from build123d import *

# Parameters (mm, degrees)
EXTRUDE_1_DEPTH     = 5.5
FILLET_2_R          = 5
SKETCH_5_R          = 0.75
CUT_EXTRUDE_3_DEPTH = 133.967101194
SKETCH_6_R          = 1.05
CUT_EXTRUDE_4_DEPTH = 133.967101194
SKETCH_7_R          = 1.05
CUT_EXTRUDE_5_DEPTH = 133.967101194
FILLET_3_R          = 3
FILLET_4_R          = 10
SKETCH_8_W          = 5.5
SKETCH_8_H          = 5.5
CUT_EXTRUDE_6_DEPTH = 133.967101194
SKETCH_9_R          = 1.05
CUT_EXTRUDE_7_DEPTH = 133.967101194
SKETCH_10_W         = 5.5
SKETCH_10_H         = 100
CUT_EXTRUDE_8_DEPTH = 133.967101194


with BuildPart() as part:
    # ｽｹｯﾁ1 → ﾎﾞｽ - 押し出し1 (new body)
    with BuildSketch(Plane.XY):
        with BuildLine():
            Line((19, 125), (-41, 125))
            Line((-41, 125), (-41, 111))
            Line((-41, 111), (-28, 95))
            Line((-28, 95), (-19, 95))
            Line((-19, 95), (-19, 56.216441442))
            ThreePointArc((-19, 56.216441442), (-31.652114797, 51.899926796), (-45, 51.163538212))
            Line((-45, 51.163538212), (-45, 48.163538212))
            Line((-45, 48.163538212), (-19, 48.163538212))
            Line((-19, 48.163538212), (-19, 23.216373532))
            ThreePointArc((-19, 23.216373532), (0, -30), (19, 23.216373532))
            Line((19, 23.216373532), (19, 125))
        make_face()
    extrude(amount=EXTRUDE_1_DEPTH)

    # ﾌｨﾚｯﾄ2
    fillet_2_edges = [part.edges().sort_by_distance(p)[0] for p in [
        (-19, 95, 2.75),
    ]]
    fillet(fillet_2_edges, radius=FILLET_2_R)

    # ｽｹｯﾁ5 → ｶｯﾄ - 押し出し3 (cut, through all)
    with BuildSketch(Plane.XY.offset(5.5)):
        with Locations((14.45, 0)):
            Circle(SKETCH_5_R)
        with Locations((-14.45, 0)):
            Circle(SKETCH_5_R)
    extrude(amount=-CUT_EXTRUDE_3_DEPTH, mode=Mode.SUBTRACT)

    # ｽｹｯﾁ6 → ｶｯﾄ - 押し出し4 (cut, through all)
    with BuildSketch(Plane.XY.offset(5.5)):
        with Locations((-24.425038206, -12.880897043)):
            Circle(SKETCH_6_R)
        with Locations((-21.701843031, -17.074249883)):
            Circle(SKETCH_6_R)
        with Locations(Location((24.425038206, -12.880897043, 0), (0, 0, 180))):
            Circle(SKETCH_6_R)
        with Locations(Location((21.701843031, -17.074249883, 0), (0, 0, 180))):
            Circle(SKETCH_6_R)
    extrude(amount=-CUT_EXTRUDE_4_DEPTH, mode=Mode.SUBTRACT)

    # ｽｹｯﾁ7 → ｶｯﾄ - 押し出し5 (cut, through all)
    with BuildSketch(Plane.XY.offset(5.5)):
        with Locations((-21.9, 100)):
            Circle(SKETCH_7_R)
        with Locations((-35.6, 110.5)):
            Circle(SKETCH_7_R)
    extrude(amount=-CUT_EXTRUDE_5_DEPTH, mode=Mode.SUBTRACT)

    # ﾌｨﾚｯﾄ3
    fillet_3_edges = [part.edges().sort_by_distance(p)[0] for p in [
        (-28, 95, 2.75),
    ]]
    fillet(fillet_3_edges, radius=FILLET_3_R)

    # ﾌｨﾚｯﾄ4
    fillet_4_edges = [part.edges().sort_by_distance(p)[0] for p in [
        (-19, 48.163538212, 2.75),
    ]]
    fillet(fillet_4_edges, radius=FILLET_4_R)

    # ｽｹｯﾁ8 → ｶｯﾄ - 押し出し6 (cut, through all)
    with BuildSketch(Plane.XY.offset(5.5)):
        with Locations((12.75, 112.25)):
            Rectangle(SKETCH_8_W, SKETCH_8_H)
        with Locations((-19.75, 112.25)):
            Rectangle(SKETCH_8_W, SKETCH_8_H)
        with Locations((12.75, 81.75)):
            Rectangle(SKETCH_8_W, SKETCH_8_H)
    extrude(amount=-CUT_EXTRUDE_6_DEPTH, mode=Mode.SUBTRACT)

    # ｽｹｯﾁ9 → ｶｯﾄ - 押し出し7 (cut, through all)
    with BuildSketch(Plane.XY.offset(5.5)):
        with Locations((16, 25)):
            Circle(SKETCH_9_R)
        with Locations((16, 29)):
            Circle(SKETCH_9_R)
        with Locations((16, 33)):
            Circle(SKETCH_9_R)
        with Locations((16, 37)):
            Circle(SKETCH_9_R)
        with Locations((16, 41)):
            Circle(SKETCH_9_R)
        with Locations((16, 45)):
            Circle(SKETCH_9_R)
        with Locations((16, 49)):
            Circle(SKETCH_9_R)
        with Locations((16, 53)):
            Circle(SKETCH_9_R)
        with Locations((16, 57)):
            Circle(SKETCH_9_R)
        with Locations(Location((-16, 57, 0), (0, 0, 180))):
            Circle(SKETCH_9_R)
        with Locations(Location((-16, 53, 0), (0, 0, 180))):
            Circle(SKETCH_9_R)
        with Locations(Location((-16, 49, 0), (0, 0, 180))):
            Circle(SKETCH_9_R)
        with Locations(Location((-16, 45, 0), (0, 0, 180))):
            Circle(SKETCH_9_R)
        with Locations(Location((-16, 41, 0), (0, 0, 180))):
            Circle(SKETCH_9_R)
        with Locations(Location((-16, 37, 0), (0, 0, 180))):
            Circle(SKETCH_9_R)
        with Locations(Location((-16, 33, 0), (0, 0, 180))):
            Circle(SKETCH_9_R)
        with Locations(Location((-16, 29, 0), (0, 0, 180))):
            Circle(SKETCH_9_R)
        with Locations(Location((-16, 25, 0), (0, 0, 180))):
            Circle(SKETCH_9_R)
    extrude(amount=-CUT_EXTRUDE_7_DEPTH, mode=Mode.SUBTRACT)

    # ｽｹｯﾁ10 → ｶｯﾄ - 押し出し8 (cut, through all)
    with BuildSketch(Plane.XY.offset(5.5)):
        with Locations((0, 75)):
            Rectangle(SKETCH_10_W, SKETCH_10_H)
    extrude(amount=-CUT_EXTRUDE_8_DEPTH, mode=Mode.SUBTRACT)


solid = part.part
Geometry: final body of the model. Coordinates: model frame, mm. A direction names the side the tool comes from. Give positions to 0.01 mm unless a question says otherwise; leave off trailing zeros. Write each loop counter-clockwise with the first axis right and the second up, starting at its lowest first coordinate (ties: lowest second). Pieces come first, ordered by that corner, then holes. Notation, with made-up numbers: (23.25, 25) -> (81.25, 25) arc R11 ccw to (81.25, 44) -> close; hole circle Ø11 at (78, 72). An arc over 180 degrees is marked (long way). Answer in a Markdown table with one row per item.
(1) Section query A-A on x = -31.5. Return loops of the section in (y, z).
Answers below:
| item | result |
|---|---|
| outline | (48.16, 0) -> (51.93, 0) -> (51.93, 5.5) -> (48.16, 5.5) -> close; (99.31, 0) -> (125, 0) -> (125, 5.5) -> (99.31, 5.5) -> close |
(2) Set-up query: faces 5 (the flat face through (10, 82, 3)), 6 (the flat face through (-19, 31, 3)), 7 (the flat face through (2.75, 74, 3)), 8 (the flat face through (-41, 118, 3)), 9 (the flat face through (-45, 50, 3)). Return all of +Z, -Z, +X, -X, +Y, -Y with unobstructed straight access to the full face (end or side cutting, diameter ignored); none if empty.
Answers below:
| item | result |
|---|---|
| face 5 | +Z, -Z |
| face 6 | +Z, -Z, -X |
| face 7 | +Z, -Z, +Y |
| face 8 | +Z, -Z, -X, +Y |
| face 9 | +Z, -Z, -X, +Y, -Y |
(3) Draft query along Y for faces 1 (the flat face through (11, 125, 3)), 2 (the flat face through (-20, 115, 3)), 3 (the flat face through (-8, 49, 5.5)), 4 (the flat face through (13, 109.5, 3)). Return one class per face: +Y half, -Y half, draft (parallel to the pull), parting line (faces both ways), or undercut.
Answers below:
| item | result |
|---|---|
| face 1 | +Y half |
| face 2 | undercut |
| face 3 | draft |
| face 4 | undercut |
(4) Section query C-C on x = -1. Return loops of the section in (y, z).
Answers below:
| item | result |
|---|---|
| outline | (-29.98, 0) -> (25, 0) -> (25, 5.5) -> (-29.98, 5.5) -> close |
(5) Section query B-B on z = 4. State how many separate pieces and enclosed holes the cut face has, then the cut area to 3 significant figures.
Answers below:
| item | result |
|---|---|
| separate pieces | 1 |
| enclosed holes | 29 |
| area | 6,490 mm^2 |
(6) Pin query (flat end, axial travel): pin 1 (1.3 mm diameter, centred on x = -16, y = 53, fed in from +Z); pin 2 (8 mm diameter, centred on x = -2.5, y = 96.5, fed in from -Z); pin 3 (3 mm diameter, centred on y = 60.5, z = 2, fed in from +X); pin 4 (3 mm diameter, centred on y = 120, z = 2, fed in from -X). Return the tip coordinate at first contact, or that it passes through.
Answers below:
| item | result |
|---|---|
| pin 1 | through |
| pin 2 | z = 0 |
| pin 3 | x = 19 |
| pin 4 | x = -41 |
(7) Ray query, line 1 along X through (y, z) = (83, 4.65); line 2 along X through (y, z) = (-18, 4.9); line 3 along X through (y, z) = (118, 4.8). Return the intervals inside material, ascending. Write a range as [from, to].
Answers below:
| item | result |
|---|---|
| line 1 | [-19, -2.75], [2.75, 10], [15.5, 19] |
| line 2 | [-24, -22.2], [-21.21, 21.21], [22.2, 24] |
| line 3 | [-41, -2.75], [2.75, 19] |
